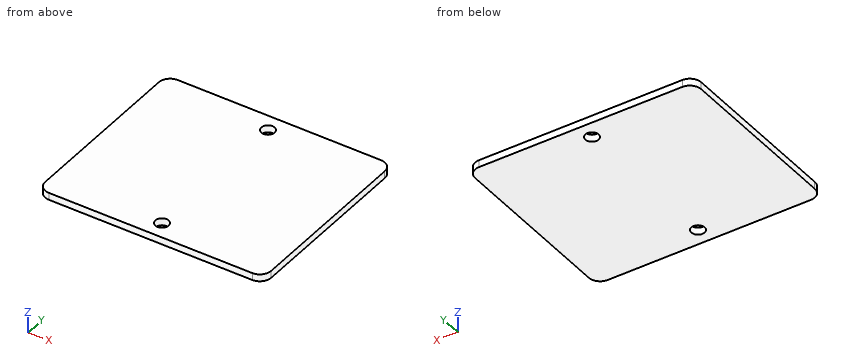
Autodesk Fusion 360 part; units mm, degrees
sketch "Sketch1" plane through (0, 0, 0) normal (0, 0, 1) x (1, 0, 0)
  line L0 (0, 0) -> (50.8, 0)
  line L1 (50.8, 0) -> (50.8, 43.18)
  line L2 (50.8, 43.18) -> (0, 43.18)
  line L3 (0, 43.18) -> (0, 0)
  line L4 (25.4, 43.18) -> (25.4, 0) construction
  line L5 (0, 21.59) -> (50.8, 21.59) construction
  circle A0 centre (25.4, 39.37) radius 1.5
  circle A1 centre (25.4, 3.81) radius 1.5
  dimension "d1" = 50.8
  dimension "d2" = 43.18
  dimension "d3" = 3
  dimension "d4" = 3
  dimension "d5" = 17.78
  dimension "d6" = 35.56
extrude "Extrude1" add sketch "Sketch1" along normal blind 1.6
fillet "Fillet1" radius 2.54 4 edges at (50.8, 0, 0.8) (50.8, 43.18, 0.8) (0, 0, 0.8) (0, 43.18, 0.8)
Verification items for the finished model (mm, model axes). Round coordinates to 2 decimals unless told otherwise and drop trailing zeros. Write each loop counter-clockwise with the first axis right and the second up, starting at its lowest first coordinate (ties: lowest second). Pieces come first, ordered by that corner, then holes.
(1) Material ranges on line 1 (Y direction, x = 25.4, z = 0.65); line 2 (X direction, y = 3, z = 0.85); line 3 (X direction, y = 2, z = 0.9), recorded low to high.
Returned:
line 1: y = 0 to 2.31, 5.31 to 37.87, 40.87 to 43.18
line 2: x = 0 to 24.14, 26.66 to 50.8
line 3: x = 0.06 to 50.74
(2) Section check B-B (x = 25.4). Enter the section's corners in (y, z).
Returned:
outline: (0, 0) - (2.31, 0) - (2.31, 1.6) - (0, 1.6) - close; (5.31, 0) - (37.87, 0) - (37.87, 1.6) - (5.31, 1.6) - close; (40.87, 0) - (43.18, 0) - (43.18, 1.6) - (40.87, 1.6) - close
(3) Section check A-A (y = 3.81). Enter the section's corners in (x, z), plus the area to 3 significant figures.
Returned:
outline: (0, 0) - (23.9, 0) - (23.9, 1.6) - (0, 1.6) - close; (26.9, 0) - (50.8, 0) - (50.8, 1.6) - (26.9, 1.6) - close
area: 76.5 mm2
